Design review of the part built by this model. Coordinates are the model's own, in mm. Face numbers are marked on the shaded views. Coordinates: 2 decimals unless noted, no trailing zeros. Loops run counter-clockwise (first coordinate to the right, second up) from the corner with the lowest first, then second, coordinate; pieces in that order, holes last. Notation, with made-up numbers: (16.25, -17.5) -> (47.25, -17.5) arc R12 cw to (47.25, -6.5) -> close; hole circle Ø10 at (-22, 74.25). An arc over 180 degrees is marked (long way). One line per item, written item: value. Start each with the question number.
1. Draft analysis for pull direction Y (two halves, no side actions). For the marked faces 1, 2 and 3, state which applies: pulls with the +Y half, pulls with the -Y half, needs draft (parallel to the pull), parting line crosses it, or undercut.
2. For probe 1 along Y at (x, z) = (0.25, -10.5); probe 2 along Y at (x, z) = (0.75, 7); probe 3 along X at (y, z) = (-67, -1), list the stretches that pass through material, from the lowest coordinate up.
3. Add section A-A on y = -123.7. Write out the cut boundary in (x, z), plus the area to 3 significant figures.
4. Add section C-C on y = -23.5. Write out the cut boundary in (x, z), plus the area to 3 significant figures.
5. Insertion check: pin 1 (3.5 mm diameter, centred on x = 0, y = -123.7, fed in from +Z); pin 2 (1.5 mm diameter, centred on x = 3, z = 12.5, fed in from +Y); pin 3 (6.5 mm diameter, centred on x = 0, y = -67.1, fed in from +Z); pin 4 (1 mm diameter, centred on x = -4, z = -9.5, fed in from -Y). Each pin has a flat end and moves straight along its axis. Give the tip position at first contact, or say it passes through.
6. Add section B-B on z = 14.5. Write out the cut boundary in (x, y), plus the area to 3 significant figures.
7. Add section D-D on y = -51. Write out the cut boundary in (x, z).
```python
from build123d import *

# Parameters (mm, degrees)
BOSS_EXTRUDE1_DEPTH      = 16.95
BOSS_EXTRUDE1_DEPTH_BACK = 16.95
SKETCH4_R                = 2.1


with BuildPart() as part:
    # Sketch4 → Boss-Extrude1 (new, two sides: drawn at the far end of the back side and taken through both)
    with BuildSketch(Plane.XY.offset(-BOSS_EXTRUDE1_DEPTH_BACK)):
        with BuildLine():
            ThreePointArc((-5.228730789, -121.994018072), (0, -129.2), (5.228730789, -121.994018072))
            ThreePointArc((5.228730789, -121.994018072), (1, -95.4), (5.228730789, -68.805981928))
            ThreePointArc((5.228730789, -68.805981928), (5.5, -67.1), (5.228730789, -65.394018072))
            ThreePointArc((5.228730789, -65.394018072), (1, -38.8), (5.228730789, -12.205981928))
            ThreePointArc((5.228730789, -12.205981928), (0, -5), (-5.228730789, -12.205981928))
            ThreePointArc((-5.228730789, -12.205981928), (-1, -38.8), (-5.228730789, -65.394018072))
            ThreePointArc((-5.228730789, -65.394018072), (-5.5, -67.1), (-5.228730789, -68.805981928))
            ThreePointArc((-5.228730789, -68.805981928), (-1, -95.4), (-5.228730789, -121.994018072))
        make_face()
        with Locations((0, -123.7)):
            Circle(SKETCH4_R, mode=Mode.SUBTRACT)
        with Locations((0, -10.5)):
            Circle(SKETCH4_R, mode=Mode.SUBTRACT)
        with Locations((0, -67.1)):
            Circle(SKETCH4_R, mode=Mode.SUBTRACT)
    extrude(amount=BOSS_EXTRUDE1_DEPTH + BOSS_EXTRUDE1_DEPTH_BACK)


solid = part.part
```
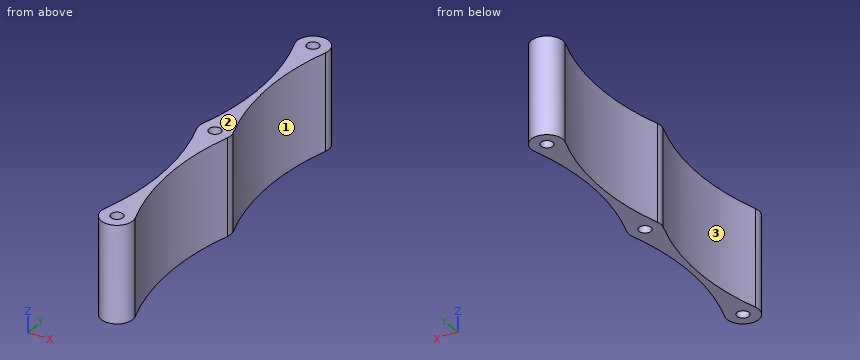
Worked answers:
1. face 1: undercut
1. face 2: needs draft
1. face 3: undercut
2. probe 1: y = -129.19 to -125.79, -121.61 to -69.19, -65.01 to -12.59, -8.41 to -5.01
2. probe 2: y = -129.15 to -125.66, -121.74 to -69.06, -65.14 to -12.46, -8.54 to -5.05
2. probe 3: x = -5.5 to -2.1, 2.1 to 5.5
3. outline: (-5.5, -16.95) -> (-2.1, -16.95) -> (-2.1, 16.95) -> (-5.5, 16.95) -> close; (2.1, -16.95) -> (5.5, -16.95) -> (5.5, 16.95) -> (2.1, 16.95) -> close
3. area: 231 mm²
4. outline: (-2.38, -16.95) -> (2.38, -16.95) -> (2.38, 16.95) -> (-2.38, 16.95) -> close
4. area: 161 mm²
5. pin 1: passes through
5. pin 2: stops at y = -5.48
5. pin 3: stops at z = 16.95
5. pin 4: stops at y = -127.94
6. outline: (-5.23, -121.99) arc R5.5 ccw (long way) to (5.23, -121.99) arc R85.74 cw to (5.23, -68.81) arc R5.5 ccw to (5.23, -65.39) arc R85.74 cw to (5.23, -12.21) arc R5.5 ccw (long way) to (-5.23, -12.21) arc R85.74 cw to (-5.23, -65.39) arc R5.5 ccw to (-5.23, -68.81) arc R85.74 cw to start; hole circle Ø4.2 at (0, -123.7); hole circle Ø4.2 at (0, -67.1); hole circle Ø4.2 at (0, -10.5)
6. area: 637 mm²
7. outline: (-1.87, -16.95) -> (1.87, -16.95) -> (1.87, 16.95) -> (-1.87, 16.95) -> close
